Can you work these out from the model? Positions are in its coordinate system, mm. Face numbers are marked on the shaded views. A direction names the side the tool comes from. Give positions to 0.01 mm unless a question says otherwise; leave off trailing zeros. Order: outer loops, then holes, each group sorted by start corner. A loop starts at its lowest first (then second) coordinate and runs counter-clockwise, first axis right, second up. Notation, with made-up numbers: (-15, 14) - (10, 14) arc R33 ccw to (10, 51) - close; hole circle Ø5 at (35.5, 3.5). An arc over 180 degrees is marked (long way). Return JSON: item names as keys, results as strings.
```python
from build123d import *

# Parameters (mm, degrees)
F0_R      = 6.35
F1_DEPTH  = 12.7
F2_W      = 20.32
F2_H      = 6.35
F3_DEPTH  = 3.175
F4_W      = 1.5748
F4_H      = 6.169682
F5_DEPTH  = 40.132
F6_R      = 4.5085
F7_DEPTH  = 14.986
F8_W      = 8.7376
F8_H      = 1.397
F9_DEPTH  = 22.86
F10_W     = 1.5748
F10_H     = 8.7376
F11_DEPTH = 37.084


with BuildPart() as f1:
    # F0 (on Front) → F1 (new body, symmetric)
    with BuildSketch(Plane.XZ):
        Circle(F0_R)
    extrude(amount=F1_DEPTH, both=True)

    # F2 (on Right) → F3 (join, symmetric)
    with BuildSketch(Plane.YZ):
        with Locations((-0.024871, -8.870569)):
            Rectangle(F2_W, F2_H)
    extrude(amount=F3_DEPTH, both=True)

    # F4 (on Front) → F5 (cut)
    with BuildSketch(Plane.XZ):
        with Locations((0.7874, -3.084841)):
            Rectangle(F4_W, F4_H)
    extrude(amount=-F5_DEPTH, mode=Mode.SUBTRACT)

    # F6 (on Front) → F7 (join)
    with BuildSketch(Plane.XZ):
        Circle(F6_R)
    extrude(amount=F7_DEPTH)

    # F8 (on Front) → F9 (cut)
    with BuildSketch(Plane.XZ):
        with Locations((0.058195, -0.036068)):
            Rectangle(F8_W, F8_H)
    extrude(amount=F9_DEPTH, mode=Mode.SUBTRACT)

    # F10 (on Front) → F11 (cut)
    with BuildSketch(Plane.XZ):
        with Locations((-0.043064, 0.016989)):
            Rectangle(F10_W, F10_H)
    extrude(amount=F11_DEPTH, mode=Mode.SUBTRACT)


solid = f1.part
```
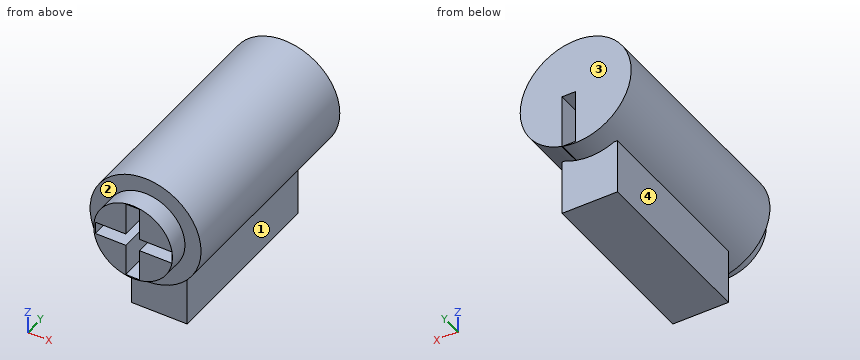
1. On a 3-axis mill with a long thin cutter (end or side, diameter ignored), from which of +Z, -Z, +X, -X, +Y, -Y can I reach the whole of each face in a straight line? I mean the marked faces 1, 2, 3 and 4. Say none if no direction works.
Checks:
{"face 1": "-Z, +X, +Y, -Y", "face 2": "-Y", "face 3": "+Z, -Z, +X, -X, +Y", "face 4": "-Z, -X, +Y, -Y"}
2. Suppose I cut it at B-B (z = -4). List the corners of the cut face in (x, y) for me, plus the area to 3 significant figures.
Checks:
{"outline": "(-4.93, -12.7) - (-2.08, -12.7) - (-2.08, -14.99) - (-0.83, -14.99) - (-0.83, 0) - (0, 0) - (0, 12.7) - (-4.93, 12.7) - close; (0.74, -14.99) - (2.08, -14.99) - (2.08, -12.7) - (4.93, -12.7) - (4.93, 12.7) - (1.57, 12.7) - (1.57, 0) - (0.74, 0) - close", "area": "216 mm^2"}
3. Suppose I cut it at A-A (y = -10.75). List the corners of the cut face in (x, z) for me, plus the area to 3 significant figures.
Checks:
{"outline": "circle Ø12.7 at (0, 0); hole (-4.31, -0.73) - (-0.83, -0.73) - (-0.83, -4.35) - (0.74, -4.35) - (0.74, -0.73) - (4.43, -0.73) - (4.43, 0.66) - (0.74, 0.66) - (0.74, 4.39) - (-0.83, 4.39) - (-0.83, 0.66) - (-4.31, 0.66) - close", "area": "103 mm^2"}
4. For pin 1 Ø4 at (y, z) = (-5.5, -2.5) entering from +X; pin 2 Ø3 at (y, z) = (-9.5, 2.5) entering from -X; pin 3 Ø1.5 at (y, z) = (-4, -2) entering from -X, each with a flat end and sliding along its axis, tell me the tip position at first contact or that it passes through.
Checks:
{"pin 1": "x = 6.33", "pin 2": "x = -6.27", "pin 3": "x = -6.23"}
5. Suppose I cut it at C-C (y = 8.25). List the corners of the cut face in (x, z) for me (3 decimals), plus the area to 3 significant figures.
Checks:
{"outline": "(-3.175, -12.046) - (3.175, -12.046) - (3.175, -5.696) - (2.808, -5.696) arc R6.35 ccw (long way) to (-2.808, -5.696) - (-3.175, -5.696) - close; hole (0, -6.17) - (1.575, -6.17) - (1.575, 0) - (0, 0) - close", "area": "155 mm^2"}
6. If I drill on L1, parallel to X at y = -4.5, z = -8.25 (3 decimals); L2, parallel to Y at x = 1.5, z = -8.5; L3, parallel to Z at x = 2.25, y = -12.5, over which ranges is the centre line in solid material (lowest first)? Write a range as [from, to].
Checks:
{"L1": "[-3.175, 3.175]", "L2": "[-10.18, 10.14]", "L3": "[-5.94, -0.73], [0.66, 5.94]"}
7. Suppose I cut it at D-D (x = -3.5). List the corners of the cut face in (y, z) for me.
Checks:
{"outline": "(-14.99, -2.84) - (-12.7, -2.84) - (-12.7, -5.3) - (12.7, -5.3) - (12.7, 5.3) - (-12.7, 5.3) - (-12.7, 2.84) - (-14.99, 2.84) - (-14.99, 0.66) - (0, 0.66) - (0, -0.73) - (-14.99, -0.73) - close"}
